```python
from build123d import *

# Parameters (mm, degrees)
SALIENTE_EXTRUIR1_DEPTH = 40
SALIENTE_EXTRUIR2_DEPTH = 5
SALIENTE_EXTRUIR3_DEPTH = 0.4


with BuildPart() as part:
    # Croquis1 → Saliente-Extruir1 (new body)
    with BuildSketch(Plane.XY):
        Polygon((-55.463005259, 96.735362128), (-111.506783676, 0.33530954), (-56.043778418, -96.400052588), (55.463005259, -96.735362128), (111.506783676, -0.33530954), (56.043778418, 96.400052588), align=None)
        Polygon((53.766067764, 92.51110391), (-53.233932236, 92.8183325), (-107, 0.30722859), (-53.766067764, -92.51110391), (53.233932236, -92.8183325), (107, -0.30722859), align=None, mode=Mode.SUBTRACT)
    extrude(amount=SALIENTE_EXTRUIR1_DEPTH)

    # Croquis2 → Saliente-Extruir2 (add)
    with BuildSketch(Plane.XY.offset(40)):
        Polygon((111.506783676, -0.33530954), (56.043778418, 96.400052588), (-55.463005259, 96.735362128), (-111.506783676, 0.33530954), (-56.043778418, -96.400052588), (55.463005259, -96.735362128), align=None)
    extrude(amount=SALIENTE_EXTRUIR2_DEPTH)

    # Croquis4 → Saliente-Extruir3 (add)
    with BuildSketch(Plane.XY.offset(45)):
        Polygon((-56.159430926, 95.537450908), (-110.810358009, 1.533220759), (-105.03688142, 1.515859468), (-53.287727951, 90.528792869), align=None)
        Polygon((-111.506783676, 0.33530954), (-110.817574962, -0.86676839), (-105.044098374, -0.884129681), (-105.733307088, 0.317948248), (-105.03688142, 1.515859468), (-110.810358009, 1.533220759), align=None)
        Polygon((-105.044098374, -0.884129681), (-110.817574962, -0.86676839), (-56.732987132, -95.197974658), (-53.831213518, -90.20667791), align=None)
        Polygon((-105.733307088, 0.317948248), (-105.044098374, -0.884129681), (-72.68406869, -0.981438798), (-73.373277404, 0.220639131), (-72.676851737, 1.418550351), (-105.03688142, 1.515859468), align=None)
        Polygon((-55.463005259, 96.735362128), (-56.159430926, 95.537450908), (-53.287727951, 90.528792869), (-52.591302284, 91.726704088), (-51.205667902, 91.722537378), (-54.077370877, 96.731195418), align=None)
        Polygon((54.658144036, 96.404219298), (-54.077370877, 96.731195418), (-51.205667902, 91.722537378), (51.756370423, 91.41292255), align=None)
        Polygon((-52.591302284, 91.726704088), (-53.287727951, 90.528792869), (-37.191985277, 62.455530537), (-36.495559609, 63.653441757), (-35.109925228, 63.649275047), (-51.205667902, 91.722537378), align=None)
        Polygon((56.043778418, 96.400052588), (54.658144036, 96.404219298), (51.756370423, 91.41292255), (53.142004804, 91.40875584), (53.831213518, 90.20667791), (56.732987132, 95.197974658), align=None)
        Polygon((53.142004804, 91.40875584), (51.756370423, 91.41292255), (35.492083414, 63.436969335), (36.877717795, 63.432802625), (37.566926509, 62.230724696), (53.831213518, 90.20667791), align=None)
        Polygon((110.817574962, 0.86676839), (56.732987132, 95.197974658), (53.831213518, 90.20667791), (105.044098374, 0.884129681), align=None)
        Polygon((72.676851737, -1.418550351), (105.03688142, -1.515859468), (105.733307088, -0.317948248), (105.044098374, 0.884129681), (72.68406869, 0.981438798), (73.373277404, -0.220639131), align=None)
        Polygon((105.03688142, -1.515859468), (110.810358009, -1.533220759), (111.506783676, -0.33530954), (110.817574962, 0.86676839), (105.044098374, 0.884129681), (105.733307088, -0.317948248), align=None)
        Polygon((53.287727951, -90.528792869), (56.159430926, -95.537450908), (110.810358009, -1.533220759), (105.03688142, -1.515859468), align=None)
        Polygon((-53.831213518, -90.20667791), (-56.732987132, -95.197974658), (-56.043778418, -96.400052588), (-54.658144036, -96.404219298), (-51.756370423, -91.41292255), (-53.142004804, -91.40875584), align=None)
        Polygon((-51.756370423, -91.41292255), (-54.658144036, -96.404219298), (54.077370877, -96.731195418), (51.205667902, -91.722537378), align=None)
        Polygon((51.205667902, -91.722537378), (54.077370877, -96.731195418), (55.463005259, -96.735362128), (56.159430926, -95.537450908), (53.287727951, -90.528792869), (52.591302284, -91.726704088), align=None)
        Polygon((35.109925228, -63.649275047), (51.205667902, -91.722537378), (52.591302284, -91.726704088), (53.287727951, -90.528792869), (37.191985277, -62.455530537), (36.495559609, -63.653441757), align=None)
        Polygon((-37.566926509, -62.230724696), (-53.831213518, -90.20667791), (-53.142004804, -91.40875584), (-51.756370423, -91.41292255), (-35.492083414, -63.436969335), (-36.877717795, -63.432802625), align=None)
        Polygon((-36.174075174, -59.834902257), (-37.566926509, -62.230724696), (-36.877717795, -63.432802625), (-35.492083414, -63.436969335), (-34.099232079, -61.041146896), (-35.48486646, -61.036980186), align=None)
        Polygon((-34.099232079, -61.041146896), (-35.492083414, -63.436969335), (35.109925228, -63.649275047), (33.7315078, -61.245119188), align=None)
        Polygon((-69.912799928, -0.989772218), (-72.68406869, -0.981438798), (-37.566926509, -62.230724696), (-36.174075174, -59.834902257), align=None)
        Polygon((33.7315078, -61.245119188), (35.109925228, -63.649275047), (36.495559609, -63.653441757), (37.191985277, -62.455530537), (35.813567849, -60.051374678), (35.117142181, -61.249285898), align=None)
        Polygon((2.074843095, -1.206244639), (0.689208714, -1.20207793), (-0.007216953, -2.399989149), (33.7315078, -61.245119188), (35.117142181, -61.249285898), (35.813567849, -60.051374678), align=None)
        Polygon((-0.696425667, -1.19791122), (-2.082060049, -1.19374451), (-36.174075174, -59.834902257), (-35.48486646, -61.036980186), (-34.099232079, -61.041146896), (-0.007216953, -2.399989149), align=None)
        Polygon((72.676851737, -1.418550351), (69.905582974, -1.410216931), (35.813567849, -60.051374678), (37.191985277, -62.455530537), align=None)
        Polygon((70.602008642, -0.212305711), (69.905582974, -1.410216931), (72.676851737, -1.418550351), (73.373277404, -0.220639131), (72.68406869, 0.981438798), (69.912799928, 0.989772218), align=None)
        Polygon((36.174075174, 59.834902257), (69.912799928, 0.989772218), (72.68406869, 0.981438798), (37.566926509, 62.230724696), align=None)
        Polygon((0.689208714, -1.20207793), (-0.696425667, -1.19791122), (-0.007216953, -2.399989149), align=None)
        Polygon((-1.385634381, 0.00416671), (-2.082060049, -1.19374451), (-0.696425667, -1.19791122), align=None)
        Polygon((-1.385634381, 0.00416671), (-0.696425667, -1.19791122), (0.689208714, -1.20207793), (1.385634381, -0.00416671), (0.696425667, 1.19791122), (-0.689208714, 1.20207793), align=None)
        Polygon((-2.074843095, 1.206244639), (-1.385634381, 0.00416671), (-0.689208714, 1.20207793), align=None)
        Polygon((0.007216953, 2.399989149), (-0.689208714, 1.20207793), (0.696425667, 1.19791122), align=None)
        Polygon((0.696425667, 1.19791122), (1.385634381, -0.00416671), (2.082060049, 1.19374451), align=None)
        Polygon((1.385634381, -0.00416671), (0.689208714, -1.20207793), (2.074843095, -1.206244639), align=None)
        Polygon((1.385634381, -0.00416671), (2.074843095, -1.206244639), (69.905582974, -1.410216931), (70.602008642, -0.212305711), (69.912799928, 0.989772218), (2.082060049, 1.19374451), align=None)
        Polygon((-70.602008642, 0.212305711), (-69.912799928, -0.989772218), (-2.082060049, -1.19374451), (-1.385634381, 0.00416671), (-2.074843095, 1.206244639), (-69.905582974, 1.410216931), align=None)
        Polygon((-35.813567849, 60.051374678), (-2.074843095, 1.206244639), (-0.689208714, 1.20207793), (0.007216953, 2.399989149), (-33.7315078, 61.245119188), (-35.117142181, 61.249285898), align=None)
        Polygon((0.007216953, 2.399989149), (0.696425667, 1.19791122), (2.082060049, 1.19374451), (36.174075174, 59.834902257), (35.48486646, 61.036980186), (34.099232079, 61.041146896), align=None)
        Polygon((35.492083414, 63.436969335), (34.099232079, 61.041146896), (35.48486646, 61.036980186), (36.174075174, 59.834902257), (37.566926509, 62.230724696), (36.877717795, 63.432802625), align=None)
        Polygon((35.492083414, 63.436969335), (-35.109925228, 63.649275047), (-33.7315078, 61.245119188), (34.099232079, 61.041146896), align=None)
        Polygon((-36.495559609, 63.653441757), (-37.191985277, 62.455530537), (-35.813567849, 60.051374678), (-35.117142181, 61.249285898), (-33.7315078, 61.245119188), (-35.109925228, 63.649275047), align=None)
        Polygon((-37.191985277, 62.455530537), (-72.676851737, 1.418550351), (-69.905582974, 1.410216931), (-35.813567849, 60.051374678), align=None)
        Polygon((-73.373277404, 0.220639131), (-72.68406869, -0.981438798), (-69.912799928, -0.989772218), (-70.602008642, 0.212305711), (-69.905582974, 1.410216931), (-72.676851737, 1.418550351), align=None)
    extrude(amount=SALIENTE_EXTRUIR3_DEPTH)


solid = part.part
```
The listing builds one solid part. Answer for the finished solid, in the listing's coordinates (mm). A direction names the side the tool comes from. Round coordinates to 2 decimals unless told otherwise and drop trailing zeros. Loops run counter-clockwise (first coordinate to the right, second up) from the corner with the lowest first, then second, coordinate; pieces in that order, holes last. Notation, with made-up numbers: (89.25, 84) - (114.25, 84) arc R17 cw to (114.25, 113) - close; hole circle Ø9 at (-13, 20). An arc over 180 degrees is marked (long way). Use one line per item in the form item = value. Start each with the question number.
1. The part is cut by section A-A on z = 15. Determine the outline of the cut face in (x, y).
2. Consider line 1 (Y direction, x = 46, z = 18.5); line 2 (Y direction, x = -45, z = 37); line 3 (Z direction, x = -76.5, y = -42). Determine where each line is inside the solid, lowest interval first. Write a range as [from, to].
3. Given pin 1 Ø6 at (y, z) = (-18.5, 37) entering from -X; pin 2 Ø1.5 at (x, z) = (43.5, 32) entering from -Y; pin 3 Ø1.5 at (x, z) = (-78.5, 16.5) entering from +Y, each flat-ended and moving along its own axis, determine where each tip first touches the part or whether it passes through.
4. A tool of negligible diameter and unlimited length cuts with its end or side. For faces 3 (the face through (79.525, -45.399, 45.197)), 4 (the face through (-80.756, -45.452, 19.72)), from which of +Z, -Z, +X, -X, +Y, -Y can it reach the whole face along a straight path? Write none if from no direction.
5. The part is cut by section C-C on y = -8.5. Determine the outline of the cut face in (x, z).
6. The part is cut by section B-B on z = 42.5. Determine the outline of the cut face in (x, y).
7. For a pull along Y with two mould halves and no side action, classify faces 1 (the face through (74, 58, 0)), 2 (the face through (-79.08, -46.17, 45.2)) as pulls with the +Y half, pulls with the -Y half, needs draft (parallel to the pull), parting line crosses it, or undercut.
8. The part is cut by section D-D on x = 76. Determine the outline of the cut face in (y, z), then the cut area to 3 significant figures.
Geometry check:
q1.outline = (-111.51, 0.34) - (-56.04, -96.4) - (55.46, -96.74) - (111.51, -0.34) - (56.04, 96.4) - (-55.46, 96.74) - close; hole (-107, 0.31) - (-53.77, -92.51) - (53.23, -92.82) - (107, -0.31) - (53.77, 92.51) - (-53.23, 92.82) - close
q2.line_1 = [-96.71, -92.8], [92.53, 96.43]
q2.line_2 = [-96.43, -92.54], [92.79, 96.7]
q2.line_3 = [40, 45]
q3.pin_1 = -102.43
q3.pin_2 = -96.7
q3.pin_3 = 58.4
q4.face_3 = +Z
q4.face_4 = -Z
q5.outline = (-106.44, 0) - (-101.95, 0) - (-101.95, 40) - (102.24, 40) - (102.24, 0) - (106.76, 0) - (106.76, 45.4) - (100.98, 45.4) - (100.98, 45) - (68.56, 45) - (68.56, 45.4) - (65.78, 45.4) - (65.78, 45) - (6.26, 45) - (6.26, 45.4) - (3.49, 45.4) - (3.49, 45) - (-3.55, 45) - (-3.55, 45.4) - (-6.33, 45.4) - (-6.33, 45) - (-65.61, 45) - (-65.61, 45.4) - (-68.37, 45.4) - (-68.37, 45) - (-100.68, 45) - (-100.68, 45.4) - (-106.44, 45.4) - close
q6.outline = (-111.51, 0.34) - (-56.04, -96.4) - (55.46, -96.74) - (111.51, -0.34) - (56.04, 96.4) - (-55.46, 96.74) - close
q7.face_1 = needs draft
q7.face_2 = undercut
q8.outline = (-61.41, 0) - (-53.65, 0) - (-53.65, 40) - (53.74, 40) - (53.74, 0) - (61.59, 0) - (61.59, 45.4) - (51.54, 45.4) - (51.54, 45) - (0.97, 45) - (0.97, 45.4) - (-1.43, 45.4) - (-1.43, 45) - (-51.46, 45) - (-51.46, 45.4) - (-61.41, 45.4) - close
q8.area = 1,250 mm^2
